from build123d import *

# Parameters (mm, degrees)
BOSS_EXTRU_1_DEPTH      = 5
ESQUISSE3_R             = 1.5
ESQUISSE3_R_2           = 0.5
ENL_V_MAT_EXTRU_1_DEPTH = 5
ESQUISSE7_W             = 5
ESQUISSE7_H             = 23
ESQUISSE7_H_2           = 5
BOSS_EXTRU_2_DEPTH      = 146
CHANFREIN1_SIZE         = 2
ENL_V_MAT_EXTRU_2_DEPTH = 146


with BuildPart() as part:
    # Esquisse6 → Boss.-Extru.1 (new body)
    with BuildSketch(Plane.XY):
        with BuildLine():
            Line((11.409894089, -29.143009992), (117.475911267, -135.20902717))
            Line((117.475911267, -135.20902717), (133.739367234, -118.945571203))
            Line((133.739367234, -118.945571203), (27.673350056, -12.879554025))
            ThreePointArc((27.673350056, -12.879554025), (-21.166010329, 19.696350392), (11.409894089, -29.143009992))
        make_face()
        with BuildLine():
            Line((-4, -23.469659936), (-4, -5.469659936))
            Line((-4, -5.469659936), (-22, -5.469659936))
            ThreePointArc((-22, -5.469659936), (-15.811388301, -17.281048237), (-4, -23.469659936))
        make_face(mode=Mode.SUBTRACT)
        with BuildLine():
            Line((-4, 2.530340064), (-4, 20.530340064))
            ThreePointArc((-4, 20.530340064), (-15.811388301, 14.341728365), (-22, 2.530340064))
            Line((-22, 2.530340064), (-4, 2.530340064))
        make_face(mode=Mode.SUBTRACT)
        with BuildLine():
            Line((4, 2.530340064), (22, 2.530340064))
            ThreePointArc((22, 2.530340064), (15.811388301, 14.341728365), (4, 20.530340064))
            Line((4, 20.530340064), (4, 2.530340064))
        make_face(mode=Mode.SUBTRACT)
        with BuildLine():
            Line((4, -5.469659936), (4, -23.469659936))
            ThreePointArc((4, -23.469659936), (15.811388301, -17.281048237), (22, -5.469659936))
            Line((22, -5.469659936), (4, -5.469659936))
        make_face(mode=Mode.SUBTRACT)
    extrude(amount=BOSS_EXTRU_1_DEPTH)

    # Esquisse3 → Enlèv. mat.-Extru.1 (cut)
    with BuildSketch(Plane.XY):
        with Locations((0, 15.030340064)):
            Circle(ESQUISSE3_R)
        with Locations((16.5, -1.469659936)):
            Circle(ESQUISSE3_R)
        with Locations((0, -17.969659936)):
            Circle(ESQUISSE3_R)
        with Locations((-16.5, -1.469659936)):
            Circle(ESQUISSE3_R)
        with Locations((0, -1.469659936)):
            Circle(ESQUISSE3_R_2)
    extrude(amount=ENL_V_MAT_EXTRU_1_DEPTH, mode=Mode.SUBTRACT)

    # Esquisse7 → Boss.-Extru.2 (add)
    with BuildSketch(Plane(origin=(126.342469219, -126.342469219, 0), x_dir=(0, 0, -1), z_dir=(0.7071067811865442, -0.7071067811865508, 0))):
        with Locations((-2.5, -1.039206507)):
            Rectangle(ESQUISSE7_W, ESQUISSE7_H)
        with Locations((2.5, -1.039206507)):
            Rectangle(ESQUISSE7_W, ESQUISSE7_H_2)
    extrude(amount=-BOSS_EXTRU_2_DEPTH)

    # Chanfrein1
    chanfrein1_edges = [part.edges().sort_by_distance(p)[0] for p in [
        (80.706358645, -65.912562614, 5),
        (-21.166010329, 19.696350392, 5),
        (64.442902678, -82.176018581, 5),
    ]]
    chamfer(chanfrein1_edges, length=CHANFREIN1_SIZE)

    # Esquisse8 → Enlèv. mat.-Extru.2 (cut)
    with BuildSketch(Plane.XY.offset(5)):
        Polygon((120.304338392, -125.309532234), (123.839872298, -121.773998328), (122.425658735, -120.359784766), (118.890124829, -123.895318671), align=None)
    extrude(amount=-ENL_V_MAT_EXTRU_2_DEPTH, mode=Mode.SUBTRACT)


solid = part.part
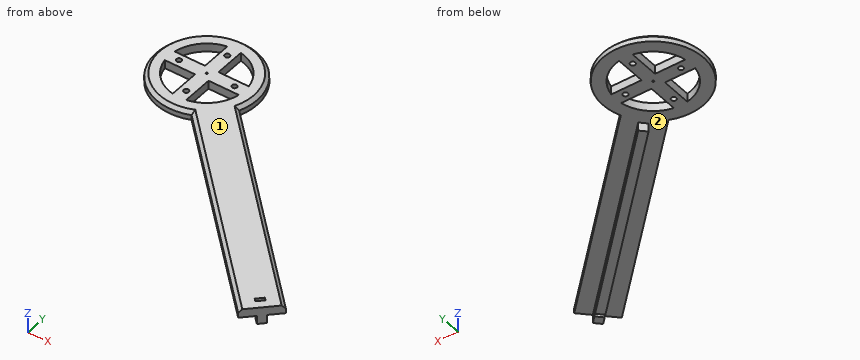
Design review of the part built by this model. Coordinates are the model's own, in mm. Face numbers are marked on the shaded views. A direction names the side the tool comes from. Coordinates: 2 decimals unless noted, no trailing zeros. Loops run counter-clockwise (first coordinate to the right, second up) from the corner with the lowest first, then second, coordinate; pieces in that order, holes last.
Item 1: Add section C-C (y = 11.5). Give the number of separate pieces and of enclosed holes in the cut face, and give its area (3 significant figures).
Completed:
separate pieces: 3
enclosed holes: 0
area: 123 mm2
Item 2: Add section A-A (z = -3). Write out the cut boundary in (x, y).
Completed:
outline: (20.6, -25.61) - (118.89, -123.9) - (122.43, -120.36) - (24.14, -22.07) - close; (120.3, -125.31) - (123.84, -128.85) - (127.38, -125.31) - (123.84, -121.77) - close
Item 3: For the marked faces 1 and 2, list the 3-axis set-ups (+Z, -Z, +X, -X, +Y, -Y) from which the entire face can be reached by the end or side of a thin tool; tool diameter is ignored.
Completed:
face 1: +Z, +X, -X, +Y, -Y
face 2: -Z
Item 4: Wall thickness on L1, parallel to Y at x = 0, z = 2.2; L2, parallel to Y at x = 16.5, z = 3.25; L3, parallel to Z at x = 54, y = -65: over which ranges is each line inside the solid? List them lowest first.
Completed:
L1: y = -31.4 to -19.47, -16.47 to -1.97, -0.97 to 13.53, 16.53 to 28.46
L2: y = -33.88 to -16.56, -5.47 to -2.97, 0.03 to 2.53, 13.62 to 23.21
L3: z = 0 to 5
Item 5: Add section B-B (x = 55). Write out the cut boundary in (y, z), and give its area (3 significant figures).
Completed:
outline: (-72.73, 0) - (-60.01, 0) - (-60.01, -5) - (-52.93, -5) - (-52.93, 0) - (-40.21, 0) - (-40.21, 3) - (-43.03, 5) - (-69.9, 5) - (-72.73, 3) - close
area: 192 mm2
Item 6: Add section D-D (y = -73). Write out the cut boundary in (x, z).
Completed:
outline: (55.27, 0) - (67.99, 0) - (67.99, -5) - (75.07, -5) - (75.07, 0) - (87.79, 0) - (87.79, 3) - (84.97, 5) - (58.1, 5) - (55.27, 3) - close
Item 7: Clearance check with flat-ended pins moving along their axes: pin 1 (1 mm diameter, centred on y = -22, z = 0, fed in from +X); pin 2 (4 mm diameter, centred on x = -10, z = 2, fed in from -Y); pin 3 (2 mm diameter, centred on x = 86, z = 2.5, fed in from +Y); pin 4 (2.5 mm diameter, centred on x = -16.5, y = -1.47, fed in from +Z). State where each tip first meets the part, or that it passes through.
Completed:
pin 1: stops at x = 37.29
pin 2: stops at y = -30.31
pin 3: stops at y = -70.21
pin 4: passes through
